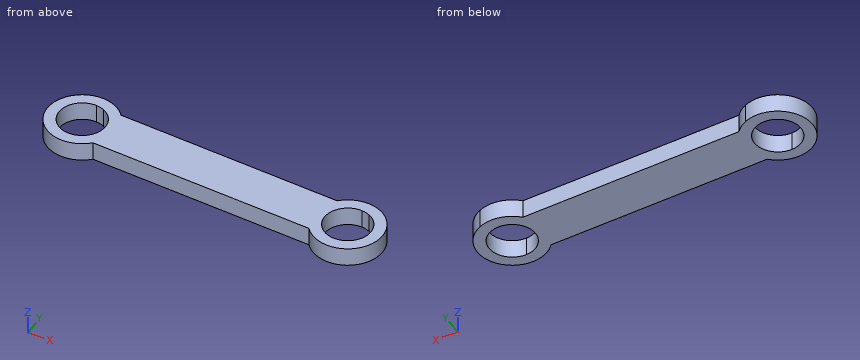
from build123d import *

# Parameters (mm, degrees)
BOSS_EXTRUDE1_DEPTH = 4


with BuildPart() as part:
    # Sketch1 → Boss-Extrude1 (new body)
    with BuildSketch(Plane(origin=(0, 0, 0), x_dir=(0.431181775, 0.902265081, 0), z_dir=(0, 0, 1))):
        with BuildLine():
            ThreePointArc((-30.032895054, 31.515538639), (-26.144357712, 35.193408701), (-20.794099729, 35.342372963))
            Line((-20.794099729, 35.342372963), (-39.476574827, 80.445857725))
            ThreePointArc((-39.476574827, 80.445857725), (-43.365112169, 76.767987664), (-48.715370152, 76.619023401))
            Line((-48.715370152, 76.619023401), (-30.032895054, 31.515538639))
        make_face()
        with BuildLine():
            ThreePointArc((-48.715370152, 76.619023401), (-43.365112169, 76.767987664), (-39.476574827, 80.445857725))
            Line((-39.476574827, 80.445857725), (-41.615840249, 85.610501319))
            ThreePointArc((-41.615840249, 85.610501319), (-41.331311509, 84.672535768), (-41.235237911, 83.697084158))
            ThreePointArc((-41.235237911, 83.697084158), (-45.259786301, 78.793157756), (-50.854635574, 81.783666996))
            Line((-50.854635574, 81.783666996), (-48.715370152, 76.619023401))
        make_face()
        with BuildLine():
            Line((-41.615840249, 85.610501319), (-39.476574827, 80.445857725))
            ThreePointArc((-39.476574827, 80.445857725), (-38.922920456, 82.029746929), (-38.735237911, 83.697084158))
            ThreePointArc((-38.735237911, 83.697084158), (-50.573959393, 89.814722256), (-48.715370152, 76.619023401))
            Line((-48.715370152, 76.619023401), (-50.854635574, 81.783666996))
            ThreePointArc((-50.854635574, 81.783666996), (-48.148655073, 88.31648182), (-41.615840249, 85.610501319))
        make_face()
        with BuildLine():
            Line((-20.794099729, 35.342372963), (-18.654834307, 30.177729369))
            ThreePointArc((-18.654834307, 30.177729369), (-18.370305568, 29.239763817), (-18.27423197, 28.264312207))
            ThreePointArc((-18.27423197, 28.264312207), (-22.298780359, 23.360385805), (-27.893629632, 26.350895045))
            Line((-27.893629632, 26.350895045), (-30.032895054, 31.515538639))
            ThreePointArc((-30.032895054, 31.515538639), (-24.941569198, 20.951994752), (-15.77423197, 28.264312207))
            ThreePointArc((-15.77423197, 28.264312207), (-17.156593871, 32.603033689), (-20.794099729, 35.342372963))
        make_face()
        with BuildLine():
            ThreePointArc((-27.893629632, 26.350895045), (-25.187649131, 32.883709869), (-18.654834307, 30.177729369))
            Line((-18.654834307, 30.177729369), (-20.794099729, 35.342372963))
            ThreePointArc((-20.794099729, 35.342372963), (-26.144357712, 35.193408701), (-30.032895054, 31.515538639))
            Line((-30.032895054, 31.515538639), (-27.893629632, 26.350895045))
        make_face()
    extrude(amount=BOSS_EXTRUDE1_DEPTH)


solid = part.part
Geometry check sheet. Reference: the model listing, model coordinates, mm. Give positions to 0.01 mm unless a question says otherwise; leave off trailing zeros. Loops run counter-clockwise (first coordinate to the right, second up) from the corner with the lowest first, then second, coordinate; pieces in that order, holes last.
(1) Section check B-B on z = 0.65. Record the cut outline in (x, y) (3 decimals), then the cut area to 3 significant figures.
From the geometry:
outline: (-90.136, -10.917) - (-41.385, -13.509) arc R7.5 ccw (long way) to (-40.854, -3.523) - (-89.605, -0.932) arc R7.5 ccw (long way) to start; hole circle Ø10 at (-95.453, -5.628); hole circle Ø10 at (-35.537, -8.812)
area: 658 mm2
(2) Section check D-D on x = -77.5. Record the cut outline in (y, z), then the cut area to 3 significant figures.
From the geometry:
outline: (-11.59, 0) - (-1.57, 0) - (-1.57, 4) - (-11.59, 4) - close
area: 40.1 mm2
(3) Section check A-A on y = -7. Record the cut outline in (x, z).
From the geometry:
outline: (-102.83, 0) - (-100.26, 0) - (-100.26, 4) - (-102.83, 4) - close; (-90.64, 0) - (-40.2, 0) - (-40.2, 4) - (-90.64, 4) - close; (-30.88, 0) - (-28.26, 0) - (-28.26, 4) - (-30.88, 4) - close
(4) Section check C-C on x = -97. Record the cut outline in (y, z).
From the geometry:
outline: (-12.97, 0) - (-10.38, 0) - (-10.38, 4) - (-12.97, 4) - close; (-0.87, 0) - (1.71, 0) - (1.71, 4) - (-0.87, 4) - close
(5) Thickness scan on L1, parallel to X at y = -7.5, z = 3.65; L2, parallel to X at y = -7, z = 1.25; L3, parallel to Y at x = -32, z = 3.65. Record the ranges inside material, lowest first.
From the geometry:
L1: x = -102.72 to -100.09, -90.82 to -40.36, -30.71 to -28.15
L2: x = -102.83 to -100.26, -90.64 to -40.2, -30.88 to -28.26
L3: y = -15.43 to -12.35, -5.28 to -2.2
